```python
from build123d import *

# Parameters (mm, degrees)
SKETCH1_W                 = 44.45
SKETCH1_H                 = 38.1
BOSS_EXTRUDE1_DEPTH       = 3.175
SKETCH2_W                 = 25.4
SKETCH2_H                 = 25.4
CUT_EXTRUDE1_DEPTH        = 3.175
F_4_CLEARANCE_HOLE1_D     = 3.2639
F_4_CLEARANCE_HOLE1_DEPTH = 10.16
F_4_CLEARANCE_HOLE1_TIP   = 0.980574487
FILLET1_R                 = 2.54


with BuildPart() as part:
    # Sketch1 → Boss-Extrude1 (new body)
    with BuildSketch(Plane(origin=(0, 0, 0), x_dir=(1, 0, 0), z_dir=(0, 1, 0))):
        Rectangle(SKETCH1_W, SKETCH1_H)
    extrude(amount=BOSS_EXTRUDE1_DEPTH)

    # Sketch2 → Cut-Extrude1 (cut)
    with BuildSketch(Plane(origin=(0, 3.175, 0), x_dir=(1, 0, 0), z_dir=(0, 1, 0))):
        Rectangle(SKETCH2_W, SKETCH2_H)
    extrude(amount=-CUT_EXTRUDE1_DEPTH, mode=Mode.SUBTRACT)

    # #4 Clearance Hole1
    with Locations(Plane(origin=(0, 3.175, 0), x_dir=(1, 0, 0), z_dir=(0, 1, 0))):
        with Locations((-17.78, 0), (17.78, 0)):
            Hole(F_4_CLEARANCE_HOLE1_D / 2, depth=F_4_CLEARANCE_HOLE1_DEPTH)
            with Locations((0, 0, -(F_4_CLEARANCE_HOLE1_DEPTH + F_4_CLEARANCE_HOLE1_TIP / 2))):  # 118° drill point
                Cone(0, F_4_CLEARANCE_HOLE1_D / 2, F_4_CLEARANCE_HOLE1_TIP, mode=Mode.SUBTRACT)

    # Fillet1
    fillet1_edges = [part.edges().sort_by_distance(p)[0] for p in [
        (22.225, 1.5875, 19.05),
        (-22.225, 1.5875, 19.05),
        (-22.225, 1.5875, -19.05),
        (22.225, 1.5875, -19.05),
    ]]
    fillet(fillet1_edges, radius=FILLET1_R)


solid = part.part
```
Input: part model. Units: mm. Frame: model coordinates. A direction names the side the tool comes from. Coordinates: 2 decimals unless noted, no trailing zeros. Write each loop counter-clockwise with the first axis right and the second up, starting at its lowest first coordinate (ties: lowest second). Pieces come first, ordered by that corner, then holes. Notation, with made-up numbers: (48, 27) -> (87, 27) arc R30 ccw to (87, 55) -> close; hole circle Ø9 at (11.5, -21). An arc over 180 degrees is marked (long way). Answer as a JSON object with one key per item and string values.
1. Section A-A on y = 1.1. Return the cut outline in (x, z) (3 decimals).
Result set:
{"outline": "(-22.225, -16.51) arc R2.54 ccw to (-19.685, -19.05) -> (19.685, -19.05) arc R2.54 ccw to (22.225, -16.51) -> (22.225, 16.51) arc R2.54 ccw to (19.685, 19.05) -> (-19.685, 19.05) arc R2.54 ccw to (-22.225, 16.51) -> close; hole circle Ø3.264 at (-17.78, 0); hole (-12.7, -12.7) -> (12.7, -12.7) -> (12.7, 12.7) -> (-12.7, 12.7) -> close; hole circle Ø3.264 at (17.78, 0)"}
2. First-contact query: P1, Ø3, axis at x = 17.78, z = 0, coming from the +Y side. Flat tip, straight axial feed; report the tip coordinate or a pass-through.
Result set:
{"P1": "passes through"}
3. Section B-B on x = 17.78. Return the cut outline in (y, z) (3 decimals), then the cut area to 3 significant figures.
Result set:
{"outline": "(0, -19.05) -> (3.175, -19.05) -> (3.175, -1.632) -> (0, -1.632) -> close; (0, 1.632) -> (3.175, 1.632) -> (3.175, 19.05) -> (0, 19.05) -> close", "area": "111 mm2"}
4. Section C-C on z = 0. Return the cut outline in (x, y) (3 decimals).
Result set:
{"outline": "(-22.225, 0) -> (-19.412, 0) -> (-19.412, 3.175) -> (-22.225, 3.175) -> close; (-16.148, 0) -> (-12.7, 0) -> (-12.7, 3.175) -> (-16.148, 3.175) -> close; (12.7, 0) -> (16.148, 0) -> (16.148, 3.175) -> (12.7, 3.175) -> close; (19.412, 0) -> (22.225, 0) -> (22.225, 3.175) -> (19.412, 3.175) -> close"}
5. Access query for faces 1 (the face through (-12.7, 2, 0)), 2 (the face through (-21.501, 1.61, -18.286)). Directions: +Z, -Z, +X, -X, +Y, -Y. A direction counts if a zero-diameter tool reaches every point of the face in a straight line with its end or side. Return the directions, or none.
Result set:
{"face 1": "+Y, -Y", "face 2": "-Z, -X, +Y, -Y"}
6. Material intervals for line 1 (X direction, y = 2.5, z = 11.5) (3 decimals); line 2 (Z direction, x = 17.78, y = 2.1); line 3 (Z direction, x = 4.5, y = 3), sorted ascending. Write a range as from..to.
Result set:
{"line 1": "x = -22.225..-12.7, 12.7..22.225", "line 2": "z = -19.05..-1.63, 1.63..19.05", "line 3": "z = -19.05..-12.7, 12.7..19.05"}
7. Section D-D on x = 6. Return the cut outline in (y, z) (3 decimals).
Result set:
{"outline": "(0, -19.05) -> (3.175, -19.05) -> (3.175, -12.7) -> (0, -12.7) -> close; (0, 12.7) -> (3.175, 12.7) -> (3.175, 19.05) -> (0, 19.05) -> close"}
8. Mould query, pull axis X, two halves, no side actions, for faces 3 (the face through (21.461, 1.61, 18.326)), 4 (the face through (0, 2, 19.05)), 5 (the face through (-19.337, 1.565, -0.49)). Classes: released by +X, released by -X, zero draft, split by the parting line, or undercut.
Result set:
{"face 3": "released by +X", "face 4": "zero draft", "face 5": "undercut"}
